Check sheet for the modelled part. Datum: model origin and axes. Units: mm. A direction names the side the tool comes from. Give positions to 0.01 mm unless a question says otherwise; leave off trailing zeros. Loops run counter-clockwise (first coordinate to the right, second up) from the corner with the lowest first, then second, coordinate; pieces in that order, holes last. Notation, with made-up numbers: (20, -19.75) - (60, -19.75) arc R24 cw to (60, 15.25) - close; hole circle Ø10 at (62.5, 0.25). An arc over 180 degrees is marked (long way). Answer in a Markdown table with one row per item. Add a question column.
(1) Sectioned sample at A-A on y = 13.5. Enter the section's corners in (x, z), then the cut area to 3 significant figures.
(2) Sectioned sample at C-C on y = 4.5. Enter the section's corners in (x, z), then the cut area to 3 significant figures.
(3) Thickness scan on L1, parallel to X at y = 1.2, z = 0; L2, parallel to Y at x = -2.35, z = 0. Record the ranges inside material, lowest first.
(4) Sectioned sample at B-B on y = 9.25. Enter the section's corners in (x, z).
(5) Draft check along Z on faces 6 (the face through (0.7, 0, -1.5)), 7 (the face through (2.155, 13.93, 1.268)), 8 (the face through (-1.96, 5.01, 1.11)). Enter one of: released by +Z, released by -Z, zero draft, split by the parting line, or undercut.
(6) Go/stop test with flat-tipped pins: P1, Ø1.5, axis at y = 12.5, z = -1, coming from the +X side; P2, Ø3, axis at x = 0, y = 12, coming from the -Z side; P3, Ø1.2, axis at x = 0, z = 0, coming from the -Y side. Record where each tip stops, or that it passes through.
(7) Set-up check for faces 1 (the face through (-2.155, 13.93, -1.267)), 2 (the face through (2.175, 13.93, -1.233)), 3 (the face through (0, 14, 2.5)), 4 (the face through (0, 6, 0)), 5 (the face through (-2, 9, 2)): record each of +Z, -Z, +X, -X, +Y, -Y from which the full face is reachable in a straight line by a thin tool's end or side.
from build123d import *

# Parameters (mm, degrees)
SKETCH1_R                                         = 3.25
SKETCH1_R_2                                       = 1.5
BOSS_EXTRUDE1_DEPTH                               = 6
SKETCH2_R                                         = 3.25
BOSS_EXTRUDE2_DEPTH                               = 3
BOSS_EXTRUDE3_DEPTH                               = 10
SKETCH4_OUTSIDE_W                                 = 29.504
SKETCH4_OUTSIDE_H                                 = 29.504
SKETCH4_OUTSIDE_R                                 = 2.5
CUT_EXTRUDE1_DEPTH                                = 10
CUT_EXTRUDE1_TAPER                                = 40
CSK_FOR_M2_5_FLAT_HEAD_MACHINE_SCREW1_D           = 2
CSK_FOR_M2_5_FLAT_HEAD_MACHINE_SCREW1_DEPTH       = 6
CSK_FOR_M2_5_FLAT_HEAD_MACHINE_SCREW1_CSINK_D     = 2.5
CSK_FOR_M2_5_FLAT_HEAD_MACHINE_SCREW1_CSINK_ANGLE = 90
CSK_FOR_M2_5_FLAT_HEAD_MACHINE_SCREW1_TIP         = 0.600860619
SKETCH8_R                                         = 1.5
CUT_EXTRUDE2_DEPTH                                = 4.25


with BuildPart() as part:
    # Sketch1 → Boss-Extrude1 (new body)
    with BuildSketch(Plane(origin=(0, 0, 0), x_dir=(1, 0, 0), z_dir=(0, 1, 0))):
        Circle(SKETCH1_R)
        Circle(SKETCH1_R_2, mode=Mode.SUBTRACT)
    extrude(amount=BOSS_EXTRUDE1_DEPTH)

    # Sketch2 → Boss-Extrude2 (add)
    with BuildSketch(Plane(origin=(0, 6, 0), x_dir=(1, 0, 0), z_dir=(0, 1, 0))):
        Circle(SKETCH2_R)
    extrude(amount=BOSS_EXTRUDE2_DEPTH)

    # Sketch3 → Boss-Extrude3 (add)
    with BuildSketch(Plane(origin=(0, 9, 0), x_dir=(1, 0, 0), z_dir=(0, 1, 0))):
        Polygon((2.886751346, 0), (1.443375673, 2.5), (-1.443375673, 2.5), (-2.886751346, 0), (-1.443375673, -2.5), (1.443375673, -2.5), align=None)
    extrude(amount=BOSS_EXTRUDE3_DEPTH)

    # Sketch4 outside → Cut-Extrude1 (cut)
    with BuildSketch(Plane(origin=(0, 19, 0), x_dir=(1, 0, 0), z_dir=(0, 1, 0))):
        Rectangle(SKETCH4_OUTSIDE_W, SKETCH4_OUTSIDE_H)
        Circle(SKETCH4_OUTSIDE_R, mode=Mode.SUBTRACT)
    extrude(amount=-CUT_EXTRUDE1_DEPTH, taper=CUT_EXTRUDE1_TAPER, mode=Mode.SUBTRACT)

    # CSK for M2.5 Flat Head Machine Screw1
    with Locations(Plane(origin=(0, 19, 0), x_dir=(1, 0, 0), z_dir=(0, 1, 0))):
        with Locations((0, 0)):
            CounterSinkHole(CSK_FOR_M2_5_FLAT_HEAD_MACHINE_SCREW1_D / 2, CSK_FOR_M2_5_FLAT_HEAD_MACHINE_SCREW1_CSINK_D / 2, depth=CSK_FOR_M2_5_FLAT_HEAD_MACHINE_SCREW1_DEPTH, counter_sink_angle=CSK_FOR_M2_5_FLAT_HEAD_MACHINE_SCREW1_CSINK_ANGLE)
            with Locations((0, 0, -(CSK_FOR_M2_5_FLAT_HEAD_MACHINE_SCREW1_DEPTH + CSK_FOR_M2_5_FLAT_HEAD_MACHINE_SCREW1_TIP / 2))):  # 118° drill point
                Cone(0, CSK_FOR_M2_5_FLAT_HEAD_MACHINE_SCREW1_D / 2, CSK_FOR_M2_5_FLAT_HEAD_MACHINE_SCREW1_TIP, mode=Mode.SUBTRACT)

    # Sketch8 → Cut-Extrude2 (cut, through all)
    with BuildSketch(Plane(origin=(0, 0, 0), x_dir=(0, 0, -1), z_dir=(1, 0, 0))):
        with Locations((0, 4)):
            Circle(SKETCH8_R)
    extrude(amount=-CUT_EXTRUDE2_DEPTH, mode=Mode.SUBTRACT)


solid = part.part
Reply:
| question | item | result |
|---|---|---|
| 1 | outline | (-2.89, 0) - (-1.44, -2.5) - (1.44, -2.5) - (2.89, 0) - (1.44, 2.5) - (-1.44, 2.5) - close; hole circle Ø2 at (0, 0) |
| 1 | area | 18.5 mm^2 |
| 2 | outline | (-2.93, -1.41) arc R3.25 ccw (long way) to (-2.93, 1.41) - (-0.5, 1.41) arc R1.5 cw (long way) to (-0.5, -1.41) - close |
| 2 | area | 20.7 mm^2 |
| 3 | L1 | -3.25 to -1.5, 1.5 to 3.25 |
| 3 | L2 | 0 to 2.5, 5.5 to 19 |
| 4 | outline | (-2.89, 0) - (-1.44, -2.5) - (1.44, -2.5) - (2.89, 0) - (1.44, 2.5) - (-1.44, 2.5) - close |
| 5 | face 6 | zero draft |
| 5 | face 7 | released by +Z |
| 5 | face 8 | undercut |
| 6 | P1 | x = 2.74 |
| 6 | P2 | z = -2.5 |
| 6 | P3 | y = 6 |
| 7 | face 1 | -Z, -X, +Y |
| 7 | face 2 | -Z, +X, +Y |
| 7 | face 3 | +Z, +X, -X, +Y |
| 7 | face 4 | -Y |
| 7 | face 5 | +Y |
